Autodesk Inventor part; units mm, degrees
ref_plane "MSC_PF1" through (0, 0, 0) normal (1, 0, 0) x (0, 1, 0)
ref_plane "MSC_PT1" through (0, 0, 0) normal (0, 0, -1) x (-1, 0, 0)
ref_plane "YZ Plane" through (0, 0, 0) normal (1, 0, 0) x (0, 1, 0)
sketch "Sketch1" plane through (0, 0, 0) normal (0, 1, 0) x (-1, 0, 0)
  point P0 (0, 0)
sketch "Sketch2" plane through (0, 0, 0) normal (0, 1, 0) x (-1, 0, 0)
  line L0 (-6, -20) -> (0, -20)
  line L1 (-6, -6.5) -> (-6, -20)
  line L2 (-12, -0.5) -> (-6, -6.5)
  line L3 (-12, 0) -> (-12, -0.5)
  line L4 (0, 0) -> (-12, 0)
  line L5 (0, -20) -> (0, 0)
  line L6 (0, -20) -> (0, 0)
  line L7 (0, -24) -> (0, 4)
  line L8 (2.4, 0) -> (-14.4, 0)
  dimension "d3" = 12
  dimension "d5" = 6
  dimension "d7" = 20
  dimension "ParC" = 0.5
  dimension "d22" = 0
  dimension "d23" = 0
  dimension "d43" = 45
revolve "Revolution1" add sketch "Sketch2" angle 360 about axis through (0, 0, -20) along (0, 0, -1)
sketch "Sketch3" plane through (0, 0, 0) normal (0, 0, 1) x (1, 0, 0)
  line L0 (-4, 2.3094) -> (-4, -2.3094)
  line L1 (0, 4.6188) -> (-4, 2.3094)
  line L2 (4, 2.3094) -> (0, 4.6188)
  line L3 (4, -2.3094) -> (4, 2.3094)
  line L4 (0, -4.6188) -> (4, -2.3094)
  line L5 (-4, -2.3094) -> (0, -4.6188)
  circle A0 centre (0, 0) radius 4 construction
  circle A1 centre (0, 0) radius 6 construction
  dimension "d11" = 8
  dimension "d13" = 120
  dimension "d15" = 120
extrude "Extrusion1" cut sketch "Sketch3" against normal blind 4.6
fillet "Fillet1" radius 1 1 edges at (-6, 0, -6.5)
chamfer "Chamfer1" distance 0.875 angle 45 1 edges at (-6, 0, -20) measured on face at (5.6201, 2.1011, -15.6381)
thread "Thread1"
ref_plane "MSC_PF1" through (0, 0, 0) normal (1, 0, 0) x (0, 1, 0)
ref_plane "MSC_PT1" through (0, 0, 0) normal (0, 0, -1) x (-1, 0, 0)
equation "\"d18\" = r"
equation "\"d19\" = 0.5 * PTC"
equation "\"d39\" = 0.5 * PTC"
equation "\"d3\" = 0.5 * dk"
equation "\"d5\" = 0.5 * NND"
equation "\"d7\" = NLG"
equation "\"d43\" = 0.5 * ang"
equation "\"d11\" = ParS"
equation "\"d16\" = ParT"
equation "\"NND\" = 12"
equation "\"PTC\" = 1.75"
equation "\"dk\" = 24"
equation "\"ParK\" = 6.5"
equation "\"ParS\" = 8"
equation "\"ParT\" = 4.6"
equation "\"r\" = 1"
equation "\"NLG\" = 20"
equation "\"ang\" = 90deg"
equation "\"THREADDIA\" = NND"
properties part number "DIN 7991 - M12x20" material "Steel, Mild"
Build history of the part. All positions in model axes, mm. A direction names the side the tool comes from. Give positions to 0.01 mm unless a question says otherwise; leave off trailing zeros. Order: outer loops, then holes, each group sorted by start corner. A loop starts at its lowest first (then second) coordinate and runs counter-clockwise, first axis right, second up. Notation, with made-up numbers: M 8.25,57 L 39.25,57 A9 ccw 39.25,74 Z; hole C 75.25,84.25 d11. An arc over 180 degrees is marked long. Use one line per item in the form item = value.
Q1. Pull direction X, two halves, no side cores. Call faces 1 (the flat face through (-1.97, 3.48, -2.27)), 2 (the flat face through (0, 0, -20)), 3 (the cylindrical face through (-11.99, -0.53, -0.25)): released by +X, released by -X, zero draft, split by the parting line, or undercut.
Conclusion:
face_1 = undercut
face_2 = zero draft
face_3 = split by the parting line
Q2. Which spindle directions (+Z, -Z, +X, -X, +Y, -Y) get a long thin tool onto all of the face, cutting with end or side? Do faces 4 (the flat face through (4, 0, -2)), 5 (the flat face through (5, 0, 0)), 6 (the cylindrical face through (-6, 0, -13)). Say none if no direction does.
Conclusion:
face_4 = +Z
face_5 = +Z, +X, -X, +Y, -Y
face_6 = -Z
Q3. Wall check: probe 1 along X at (y, z) = (-4, -1.5); probe 2 along Z at (x, y) = (3.5, -7.75); probe 3 along Y at (x, z) = (0, -12.75). Give the ranges that are in metal, low to high.
Conclusion:
probe_1 = -10.25 to -1.07, 1.07 to 10.25
probe_2 = -4 to 0
probe_3 = -6 to 6
Q4. Pin check, flat tips, straight feed: P1, Ø10, axis at y = -2, z = -13, coming from the -X side; P2, Ø3, axis at x = 2.5, z = -16.5, coming from the +Y side; P3, Ø4, axis at x = 3.5, z = -4.5, coming from the -Y side. Stop position of each tip, or through.
Conclusion:
P1 = -6
P2 = 5.92
P3 = -9.47
Q5. Slice it at B-B, the plane z = -5.25. Write the cut outline in (x, y).
Conclusion:
outline = C 0,0 d14.5
Q6. Slice it at A-A, the plane z = -2.75. Write the cut outline in (x, y).
Conclusion:
outline = C 0,0 d19.5; hole M -4,-2.31 L 0,-4.62 L 4,-2.31 L 4,2.31 L 0,4.62 L -4,2.31 Z
Q7. Slice it at C-C, the plane z = -13.75. Write the cut outline in (x, y).
Conclusion:
outline = C 0,0 d12
